Autodesk Inventor part; units mm, degrees
ref_plane "YZ Plane" through (0, 0, 0) normal (1, 0, 0) x (0, 1, 0)
ref_plane "XZ Plane" through (0, 0, 0) normal (0, 1, 0) x (-1, 0, 0)
ref_plane "XY Plane" through (0, 0, 0) normal (0, 0, 1) x (1, 0, 0)
sketch "Sketch1" plane through (0, 0, 0) normal (0, 1, 0) x (-1, 0, 0)
  circle A0 centre (0, 0) radius 3.81
  dimension "d0" = 7.62
extrude "Extrusion1" add sketch "Sketch1" along normal blind 44.45
sketch "Sketch2" plane through (0, 44.45, 0) normal (0, 1, 0) x (1, 0, 0)
  circle A0 centre (0, 0) radius 1.5875
  dimension "d3" = 3.175
extrude "Extrusion2" cut sketch "Sketch2" against normal blind 40.64
sketch "Sketch3" plane through (0, 0, 0) normal (0, -1, 0) x (1, 0, 0)
  line L0 (3.8861, -1.5875) -> (-3.8861, -1.5875)
  line L1 (-3.8861, -1.5875) -> (-3.8861, 1.5875)
  line L2 (-3.8861, 1.5875) -> (3.8861, 1.5875)
  line L3 (3.8861, 1.5875) -> (3.8861, -1.5875)
  line L4 (3.8861, -1.5875) -> (-3.8861, 1.5875) construction
  line L5 (-3.8861, -1.5875) -> (3.8861, 1.5875) construction
  point P0 (0, 0)
extrude "Extrusion3" add sketch "Sketch3" along normal blind 7.112
sketch "Sketch5" plane through (-3.8861, 0, 1.5875) normal (0, 0, 1) x (1, 0, 0)
  circle A0 centre (3.8861, -3.5629) radius 3.175
  point P0 (3.8861, 0)
  dimension "d16" = 6.35
extrude "Extrusion4" cut sketch "Sketch5" against normal blind 6.35
fillet "Fillet2" radius 1.5875 4 edges at (3.8861, 0, 0) (3.8861, -7.112, 0) (-3.8861, 0, 0) (-3.8861, -7.112, 0)
properties part number "cylendar2"
Source: CAD feature listing. Evaluate the final solid. Frame: model axes, mm. A direction names the side the tool comes from. Coordinates: 2 decimals unless noted, no trailing zeros. Order: outer loops, then holes, each group sorted by start corner. A loop starts at its lowest first (then second) coordinate and runs counter-clockwise, first axis right, second up. Notation, with made-up numbers: M -4.75,33 L 48.25,33 A29 cw 48.25,58 Z; hole C -25,-16.75 d2. An arc over 180 degrees is marked long. Write each question's results on one line, items separated by ' | '. Start each with the question number.
Item 1: Cut plane B-B (y = 32). Return loops of the section in (x, z) (1 decimal), and give its area (3 significant figures).
Item 2: Set-up query: faces 4 (the face through (-0.8, -0.3, -1.588)), 5 (the face through (-0.34, 24.41, 1.55)), 6 (the face through (0, 0, 2)). Return all of +Z, -Z, +X, -X, +Y, -Y with unobstructed straight access to the full face (end or side cutting, diameter ignored); none if empty.
Item 3: Cut plane A-A (x = 0). Return loops of the section in (y, z), and give its area (3 significant figures).
Item 4: Line query: probe 1 along Y at (x, z) = (0, -0.6); probe 2 along X at (y, z) = (35, 0). Output: solid intervals per line, ascending.
Item 5: Cut plane C-C (y = 2). Return loops of the section in (x, z).
Item 6: Cut plane D-D (x = -2.75). Return loops of the section in (y, z).
Item 7: First-contact query: pin 1 Ø2 at (x, y) = (-1.5, -5) entering from -Z; pin 2 Ø4 at (x, y) = (2.5, 5) entering from -Z; pin 3 Ø1 at (x, z) = (0, -1) entering from +Y; pin 4 Ø3 at (y, z) = (33.5, 0.5) entering from -X. Flat tips, straight axial feed; report the tip coordinate or a pass-through.
Item 8: Draft query along Y for faces 1 (the face through (-0.69, -6.66, 0.02)), 2 (the face through (0.83, 21.91, 3.72)), 3 (the face through (-3.41, -6.66, -0.02)). Return one class per face: pulls with the +Y half, pulls with the -Y half, needs draft (parallel to the pull), parting line crosses it, or undercut.
Checked values:
1) outline: C 0,0 d7.6; hole C 0,0 d3.2 | area: 37.7 mm2
2) face 4: -Z, +X, -X, -Y | face 5: +Y | face 6: +Z, +X, -X, -Y
3) outline: M -7.11,-1.59 L -6.74,-1.59 L -6.74,1.59 L -7.11,1.59 Z; M -0.39,-1.59 L 0,-1.59 L 0,-3.81 L 44.45,-3.81 L 44.45,-1.59 L 3.81,-1.59 L 3.81,1.59 L 44.45,1.59 L 44.45,3.81 L 0,3.81 L 0,1.59 L -0.39,1.59 Z | area: 212 mm2
4) probe 1: y = -7.11 to -6.74, -0.39 to 3.81 | probe 2: x = -3.81 to -1.59, 1.59 to 3.81
5) outline: C 0,0 d7.62
6) outline: M -7.05,-1.59 L -5.15,-1.59 L -5.15,1.59 L -7.05,1.59 Z; M -1.98,-1.59 L 0,-1.59 L 0,-2.64 L 44.45,-2.64 L 44.45,2.64 L 0,2.64 L 0,1.59 L -1.98,1.59 Z
7) pin 1: passes through | pin 2: stops at z = -3.78 | pin 3: stops at y = 3.81 | pin 4: stops at x = -3.81
8) face 1: undercut | face 2: needs draft | face 3: pulls with the -Y half
